For this review, take the finished solid that the model builds, in its own axes (mm). Give positions to 0.01 mm unless a question says otherwise; leave off trailing zeros. Write each loop counter-clockwise with the first axis right and the second up, starting at its lowest first coordinate (ties: lowest second). Pieces come first, ordered by that corner, then holes. Notation, with made-up numbers: (63.5, -15) -> (89.5, -15) arc R25 cw to (89.5, -2) -> close; hole circle Ø8 at (13, -12). An arc over 180 degrees is marked (long way). Return JSON: item names as keys, results as strings.
from build123d import *

# Parameters (mm, degrees)
SKETCH1_W                             = 1000
SKETCH1_H                             = 650
BOSS_EXTRUDE1_DEPTH                   = 6.35
SKETCH2_R                             = 9
SKETCH2_R_2                           = 4
SKETCH2_W                             = 500
SKETCH2_H                             = 200
SKETCH2_W_2                           = 450
SKETCH2_H_2                           = 250
CUT_EXTRUDE1_DEPTH                    = 6.35
F_10_CLEARANCE_HOLE1_MOUNTING_HOLES_D = 5.1054
M27_CLEARANCE_HOLE1_BUTTONS_D         = 27
F_12_0MM_DOWEL_HOLE1_SWITCHES_D       = 12
F_6_CLEARANCE_HOLE2_D                 = 3.7973


with BuildPart() as part:
    # Sketch1 → Boss-Extrude1 (new body)
    with BuildSketch(Plane.XY):
        with Locations((0, -55)):
            Rectangle(SKETCH1_W, SKETCH1_H)
    extrude(amount=BOSS_EXTRUDE1_DEPTH)

    # Sketch2 → Cut-Extrude1 (cut)
    with BuildSketch(Plane.XY):
        with Locations((300, 120)):
            Circle(SKETCH2_R)
        with Locations((250, 120)):
            Circle(SKETCH2_R)
        with Locations((200, 120)):
            Circle(SKETCH2_R)
        with Locations((-225, -251)):
            Circle(SKETCH2_R_2)
        with Locations((-225, -200)):
            Circle(SKETCH2_R_2)
        with Locations((-276, -200)):
            Circle(SKETCH2_R_2)
        with Locations((-276, -251)):
            Circle(SKETCH2_R_2)
        with Locations((150, -233)):
            Rectangle(SKETCH2_W, SKETCH2_H)
        with Locations((-175, 75)):
            Rectangle(SKETCH2_W_2, SKETCH2_H_2)
    extrude(amount=CUT_EXTRUDE1_DEPTH, mode=Mode.SUBTRACT)

    # #10 Clearance Hole1 - Mounting Holes (through all)
    with Locations(Plane(origin=(0, 0, 0), x_dir=(-1, 0, 0), z_dir=(0, 0, -1))):
        with Locations((-468.25, -354.6), (-468.25, -202.2), (-468.25, -60.2), (-468.25, 92.2), (-468.25, 244.6), (-315.85, 244.6), (-163.45, 244.6), (0, 244.6), (163.45, 244.6), (315.85, 244.6), (468.25, 244.6), (468.25, 92.2), (468.25, -354.6), (468.25, -202.2), (468.25, -60.2)):
            Hole(F_10_CLEARANCE_HOLE1_MOUNTING_HOLES_D / 2)

    # M27 Clearance Hole1 - Buttons (through all)
    with Locations(Plane(origin=(0, 0, 0), x_dir=(-1, 0, 0), z_dir=(0, 0, -1))):
        with Locations((-300, 20), (-250, 20), (-200, 20)):
            Hole(M27_CLEARANCE_HOLE1_BUTTONS_D / 2)

    # Ø12.0mm Dowel Hole1 - Switches (through all)
    with Locations(Plane(origin=(0, 0, 0), x_dir=(-1, 0, 0), z_dir=(0, 0, -1))):
        with Locations((-300, 70), (-250, 70), (-200, 70)):
            Hole(F_12_0MM_DOWEL_HOLE1_SWITCHES_D / 2)

    # #6 Clearance Hole2 (through all)
    with Locations(Plane(origin=(0, 0, 0), x_dir=(-1, 0, 0), z_dir=(0, 0, -1))):
        with Locations((412.55625, 89), (412.55625, 61)):
            Hole(F_6_CLEARANCE_HOLE2_D / 2)


solid = part.part
1. The part is to be moulded in two halves that separate along X. For faces 1 (the flat face through (-7, -50.4, 6.35)), 2 (the cylindrical face through (212.877, 24.055, 3.219)), say which applies: +X half, -X half, draft (parallel to the pull), parting line (faces both ways), or undercut.
Results found:
{"face 1": "draft", "face 2": "undercut"}
2. To check wall thickness, follow probe 1 along Y at (x, z) = (-36.5, 3.5); probe 2 along Y at (x, z) = (200, 1.5); probe 3 along X at (y, z) = (-354.6, 3.25). State the ranges of each line that lie inside material, in increasing order.
Results found:
{"probe 1": "y = -380 to -333, -133 to -50, 200 to 270", "probe 2": "y = -380 to -333, -133 to 6.5, 33.5 to 64, 76 to 111, 129 to 270", "probe 3": "x = -500 to -470.8, -465.7 to 465.7, 470.8 to 500"}
3. Add section B-B, the plane z = 2. Count the separate pieces of the cut face and the enclosed holes in it, plus the area to 3 significant figures.
Results found:
{"separate pieces": "1", "enclosed holes": "32", "area": "434,000 mm²"}
4. Add section A-A, the plane x = 32. State the section outline as (y, z) points, plus the area to 3 significant figures.
Results found:
{"outline": "(-380, 0) -> (-333, 0) -> (-333, 6.35) -> (-380, 6.35) -> close; (-133, 0) -> (-50, 0) -> (-50, 6.35) -> (-133, 6.35) -> close; (200, 0) -> (270, 0) -> (270, 6.35) -> (200, 6.35) -> close", "area": "1,270 mm²"}
5. For pin 1 (3 mm diameter, centred on x = -468.25, y = 92.2, fed in from -Z), flat-tipped, find the tip position at first contact; note if it passes through.
Results found:
{"pin 1": "passes through"}
